Here's how the part is built. I have some questions about the finished solid (model axes, mm). A direction names the side the tool comes from. Round coordinates to 2 decimals unless told otherwise and drop trailing zeros. Order: outer loops, then holes, each group sorted by start corner. A loop starts at its lowest first (then second) coordinate and runs counter-clockwise, first axis right, second up. Notation, with made-up numbers: M 6,67 L 55,67 A25 cw 55,99 Z; hole C 51,74.5 d8. An arc over 180 degrees is marked long. Use one line per item in the form item = value. Start each with the question number.
```python
from build123d import *

# Parameters (mm, degrees)
F0_R     = 7.5
F1_DEPTH = 1
F2_R     = 5
F3_DEPTH = 55
F5_R     = 1.5
F6_DEPTH = 32.501
F7_DEPTH = 48


with BuildPart() as f1:
    # F0 (on Top) → F1 (new body)
    with BuildSketch(Plane.XY):
        Circle(F0_R)
    extrude(amount=F1_DEPTH)

    # F2 (on face) → F3 (join)
    with BuildSketch(Plane.XY.offset(1)):
        Circle(F2_R)
    extrude(amount=F3_DEPTH)

    # F5 (on face) → F6 (cut, through all)
    with BuildSketch(Plane.YZ.offset(25)):
        with Locations((0, 51)):
            Circle(F5_R)
    extrude(amount=-F6_DEPTH, mode=Mode.SUBTRACT)

    # F2 (on face) → F7 (join)
    with BuildSketch(Plane.XY.offset(1)):
        Circle(F2_R)
    extrude(amount=F7_DEPTH)


solid = f1.part
```
1) If we section it at B-B on x = 0: Write out the boundary of the cut face in (y, z), then the cut area to 3 significant figures.
2) If we section it at A-A on y = 0: Write out the boundary of the cut face in (x, z), then the cut area to 3 significant figures.
3) If we section it at C-C on z = 17.5: Write out the boundary of the cut face in (x, y).
4) On a 3-axis mill with a long thin cutter (end or side, diameter ignored), from which of +Z, -Z, +X, -X, +Y, -Y can I reach the whole of each face in a straight line? I mean faces 4 (the cylindrical face through (-1.08, -4.88, 28.12)), 5 (the cylindrical face through (-7.493, 0.33, 0.493)). Say none if no direction works.
5) Will these pins go through, and if not, where does the flat tip stop? pin 1 Ø2 at (y, z) = (-2.5, 39.5) entering from +X; pin 2 Ø8 at (x, z) = (-3.5, 7.5) entering from +Y; pin 3 Ø4 at (y, z) = (0, 51) entering from +X.
6) If I drill on line 1 (Z direction, x = 2.25, y = 0); line 2 (Z direction, x = -6.5, y = -3.25); line 3 (Y direction, x = 1.25, z = 51), over which ranges is the centre line in solid material (lowest first)?
7) If we mould it in two halves opening along Z, with no side actions, what happens to faces 1 (the flat face through (0, 0, 0)), 2 (the flat face through (0, 0, 56)), 3 (the cylindrical face through (0.07, -0.325, 49.536))? For each: +Z half, -Z half, draft (parallel to the pull), parting line (faces both ways), or undercut.
8) If we section it at D-D on x = -6: Write out the boundary of the cut face in (y, z), then the cut area to 3 significant figures.
Completed:
q1.outline = M -7.5,0 L 7.5,0 L 7.5,1 L 5,1 L 5,56 L -5,56 L -5,1 L -7.5,1 Z; hole C 0,51 d3
q1.area = 558 mm²
q2.outline = M -7.5,0 L 7.5,0 L 7.5,1 L 5,1 L 5,49.5 L -5,49.5 L -5,1 L -7.5,1 Z; M -5,52.5 L 5,52.5 L 5,56 L -5,56 Z
q2.area = 535 mm²
q3.outline = C 0,0 d10
q4.face_4 = +Z
q4.face_5 = +Z, -Z
q5.pin_1 = 4.77
q5.pin_2 = 5
q5.pin_3 = 5
q6.line_1 = 0 to 49.5, 52.5 to 56
q6.line_2 = 0 to 1
q6.line_3 = -4.84 to -1.5, 1.5 to 4.84
q7.face_1 = -Z half
q7.face_2 = +Z half
q7.face_3 = undercut
q8.outline = M -4.5,0 L 4.5,0 L 4.5,1 L -4.5,1 Z
q8.area = 9.00 mm²
